For this review, take the finished solid that the model builds, in its own axes (mm). A direction names the side the tool comes from. Give positions to 0.01 mm unless a question says otherwise; leave off trailing zeros. Loops run counter-clockwise (first coordinate to the right, second up) from the corner with the lowest first, then second, coordinate; pieces in that order, holes last.
```python
from build123d import *

# Parameters (mm, degrees)
BOSS_EXTRUDE1_DEPTH      = 55
SHELL1_T                 = -5
SHELL1_THICKNESS_2_DEPTH = 4


with BuildPart() as part:
    # Sketch1 → Boss-Extrude1 (new body)
    with BuildSketch(Plane(origin=(0, 0, 0), x_dir=(1, 0, 0), z_dir=(0, 1, 0))):
        Polygon((173.205080757, 0), (86.602540378, 150), (-86.602540378, 150), (-173.205080757, 0), (-86.602540378, -150), (86.602540378, -150), align=None)
    extrude(amount=BOSS_EXTRUDE1_DEPTH)

    # Shell1
    shell1_openings = [part.faces().sort_by_distance(p)[0] for p in [
        (0, 55, 0),
    ]]
    offset(amount=SHELL1_T, openings=shell1_openings, kind=Kind.INTERSECTION)

    # Shell1 thickness 2 face (on inner face of the shell) → Shell1 thickness 2 (cut)
    with BuildSketch(Plane(origin=(0, 5, 0), x_dir=(0, 0, -1), z_dir=(0, -1, 0))):
        Polygon((-145, 83.715789032), (0, 167.431578065), (145, 83.715789032), (145, -83.715789032), (0, -167.431578065), (-145, -83.715789032), align=None)
    extrude(amount=SHELL1_THICKNESS_2_DEPTH, mode=Mode.SUBTRACT)


solid = part.part
```
Item 1: Take a section at B-B on x = 55. Give the boundary of the cut face in (y, z).
Answer:
outline: (0, -150) - (55, -150) - (55, -145) - (1, -145) - (1, 145) - (55, 145) - (55, 150) - (0, 150) - close
Item 2: Tool access review of faces 4 (the flat face through (126.16, 27.622, -71.485)), 5 (the flat face through (-129.298, 27.115, -76.05)): name each direction out of +Z, -Z, +X, -X, +Y, -Y from which nothing blocks a thin tool from reaching the whole face with its end or side.
Answer:
face 4: +Y
face 5: -Z, -X, +Y, -Y
Item 3: Take a section at A-A on y = 11.5. Give the boundary of the cut face in (x, z), and give its area (3 significant figures).
Answer:
outline: (-173.21, 0) - (-86.6, -150) - (86.6, -150) - (173.21, 0) - (86.6, 150) - (-86.6, 150) - close; hole (-167.43, 0) - (-83.72, -145) - (83.72, -145) - (167.43, 0) - (83.72, 145) - (-83.72, 145) - close
area: 5,110 mm2
Item 4: Clearance check with flat-ended pins moving along their axes: pin 1 Ø2 at (x, z) = (-110.5, 71.5) entering from +Y; pin 2 Ø6 at (y, z) = (37.5, -69.5) entering from -X; pin 3 Ø2 at (x, y) = (117, 20.5) entering from +Z. State where each tip first meets the part, or that it passes through.
Answer:
pin 1: stops at y = 1
pin 2: stops at x = -134.81
pin 3: stops at z = 99.08
Item 5: Take a section at C-C on z = -40.5. Give the boundary of the cut face in (x, y), and give its area (3 significant figures).
Answer:
outline: (-149.82, 0) - (149.82, 0) - (149.82, 55) - (144.05, 55) - (144.05, 1) - (-144.05, 1) - (-144.05, 55) - (-149.82, 55) - close
area: 923 mm2
Item 6: For L1, parallel to Z at x = -21.5, y = 36; L2, parallel to Y at x = 70.5, z = -92; L3, parallel to X at y = 24.5, z = 52, list the stretches that pass through material, from the lowest coordinate up.
Answer:
L1: z = -150 to -145, 145 to 150
L2: y = 0 to 1
L3: x = -143.18 to -137.41, 137.41 to 143.18
Item 7: The part is to be moulded in two halves that separate along X. For faces 1 (the flat face through (-1, 27, 150)), 2 (the flat face through (129.298, 27.115, 76.05)), 3 (the flat face through (-126.16, 27.622, 71.485)), say which applies: released by +X, released by -X, zero draft, split by the parting line, or undercut.
Answer:
face 1: zero draft
face 2: released by +X
face 3: undercut
